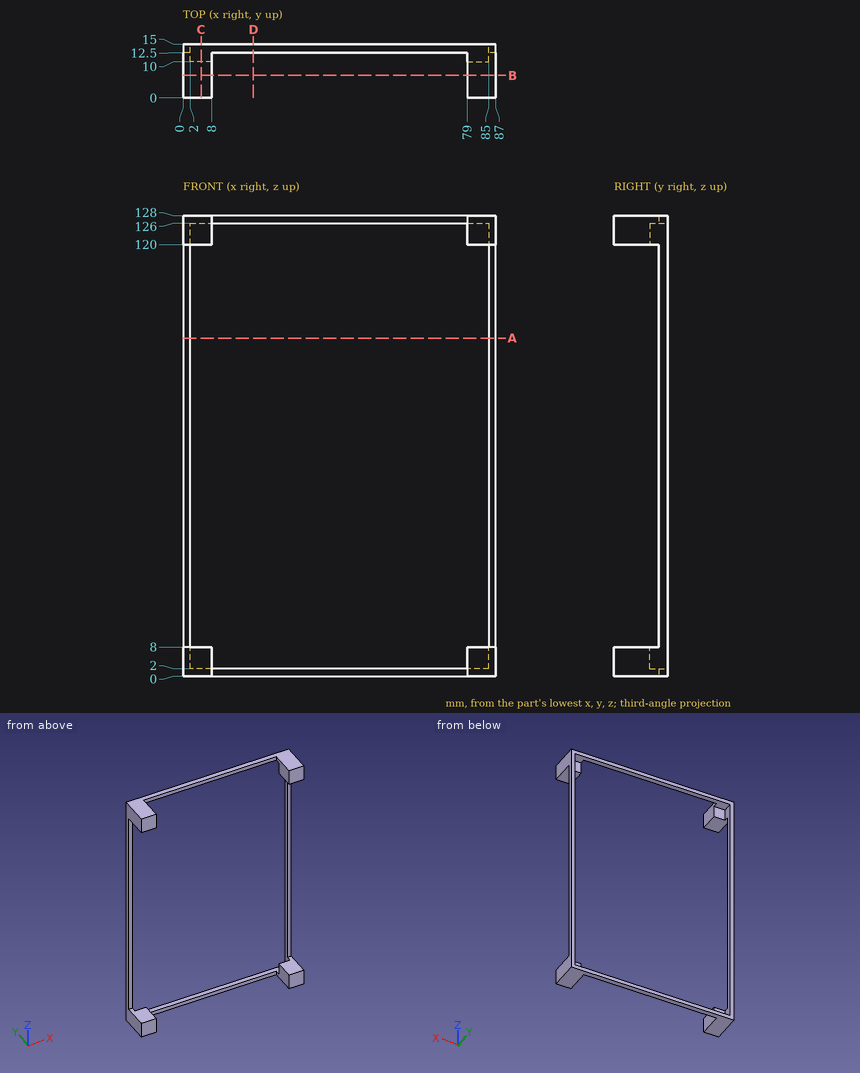
The figure shows three views and two pictorial views of one solid part (mm, origin at its lowest corner). Answer the questions. Round coordinates to 2 decimals unless told otherwise and drop trailing zeros. Order: outer loops, then holes, each group sorted by start corner. A loop starts at its lowest first (then second) coordinate and runs counter-clockwise, first axis right, second up. Notation, with made-up numbers: (-16, 23) -> (7, 23) arc R26 cw to (7, 43) -> close; hole circle Ø8 at (24, 3.5). An arc over 180 degrees is marked (long way). One line per item, written item: value.
Item 1: Given P1, Ø2, axis at x = 1, z = 89, coming from the -Y side; P2, Ø1.8, axis at x = 4.5, z = 4.5, coming from the +Y side, each flat-ended and moving along its own axis, determine where each tip first touches the part or whether it passes through.
Taken from the geometry:
P1: stops at y = 12.5
P2: stops at y = 10
Item 2: Find section D-D, the plane x = 19.5. Give the vertices of the cut face in (y, z), then the cut area to 3 significant figures.
Taken from the geometry:
outline: (12.5, 0) -> (15, 0) -> (15, 2) -> (12.5, 2) -> close; (12.5, 126) -> (15, 126) -> (15, 128) -> (12.5, 128) -> close
area: 10.0 mm2
Item 3: Straight lines are drawn through the part: L1, parallel to X at y = 13.25, z = 69; L2, parallel to X at y = 6.5, z = 120.5; L3, parallel to Z at x = 28, y = 13.75. For each, find the intervals that lie inside material, in ascending order.
Taken from the geometry:
L1: x = 0 to 2, 85 to 87
L2: x = 0 to 8, 79 to 87
L3: z = 0 to 2, 126 to 128
Item 4: Find section B-B, the plane y = 6.25. Give the vertices of the cut face in (x, z), then the cut area to 3 significant figures.
Taken from the geometry:
outline: (0, 0) -> (8, 0) -> (8, 8) -> (0, 8) -> close; (0, 120) -> (8, 120) -> (8, 128) -> (0, 128) -> close; (79, 0) -> (87, 0) -> (87, 8) -> (79, 8) -> close; (79, 120) -> (87, 120) -> (87, 128) -> (79, 128) -> close
area: 256 mm2
Item 5: Find section C-C, the plane x = 5. Give the vertices of the cut face in (y, z).
Taken from the geometry:
outline: (0, 0) -> (15, 0) -> (15, 2) -> (10, 2) -> (10, 8) -> (0, 8) -> close; (0, 120) -> (10, 120) -> (10, 126) -> (15, 126) -> (15, 128) -> (0, 128) -> close
Item 6: Find section A-A, the plane z = 94. Give the vertices of the cut face in (x, y), then the cut area to 3 significant figures.
Taken from the geometry:
outline: (0, 12.5) -> (2, 12.5) -> (2, 15) -> (0, 15) -> close; (85, 12.5) -> (87, 12.5) -> (87, 15) -> (85, 15) -> close
area: 10.0 mm2
